Answer from the drawing. Dimensions are ordinates in mm from the lowest x, y and z of the part. A direction names the side the tool comes from. Round coordinates to 2 decimals unless told otherwise and drop trailing zeros. Loops run counter-clockwise (first coordinate to the right, second up) from the corner with the lowest first, then second, coordinate; pieces in that order, holes last. Notation, with made-up numbers: (53.25, 89) - (82.25, 89) arc R9 cw to (82.25, 98) - close; hole circle Ø6 at (53.25, -17). An arc over 180 degrees is marked (long way). Answer as CSV lines item,"result". Start each with the question number.
Q1. Section C-C on z = 6 is taken. Count the separate pieces of the cut face and the enclosed holes in it, then the cut area to 3 significant figures.
Q2. Section D-D on y = 67 is taken. Write down the section's boundary in (x, z).
Q3. For the marked faces 1 and 2, determine the directions among +Z, -Z, +X, -X, +Y, -Y from which every point of the face is accessible in a straight line to the end or side of a thin tool.
Q4. Each of these flat-tipped pins is pushed along its axis until it touches: pin 1 Ø4.5 at (x, y) = (46, 8) entering from +Z; pin 2 Ø15 at (x, y) = (32.5, 38.5) entering from +Z. Where does it stop, or does it pass through?
Q5. The mould has two halves that part along X. Classify the marked faces 3, 4, 5 and 6: +X half, -X half, draft (parallel to the pull), parting line (faces both ways), or undercut.
Q6. Straight lines are drawn through the part: L1, parallel to Y at x = 46, z = 2.5; L2, parallel to Y at x = 27, z = 6.25; L3, parallel to X at y = 73, z = 3. For each, find the intervals that lie inside material, in ascending order. Write a range as [from, to].
Q7. Section B-B on y = 41 is taken. Write down the section's boundary in (x, z).
Q8. Section A-A on x = 8 is taken. Write down the section's boundary in (y, z).
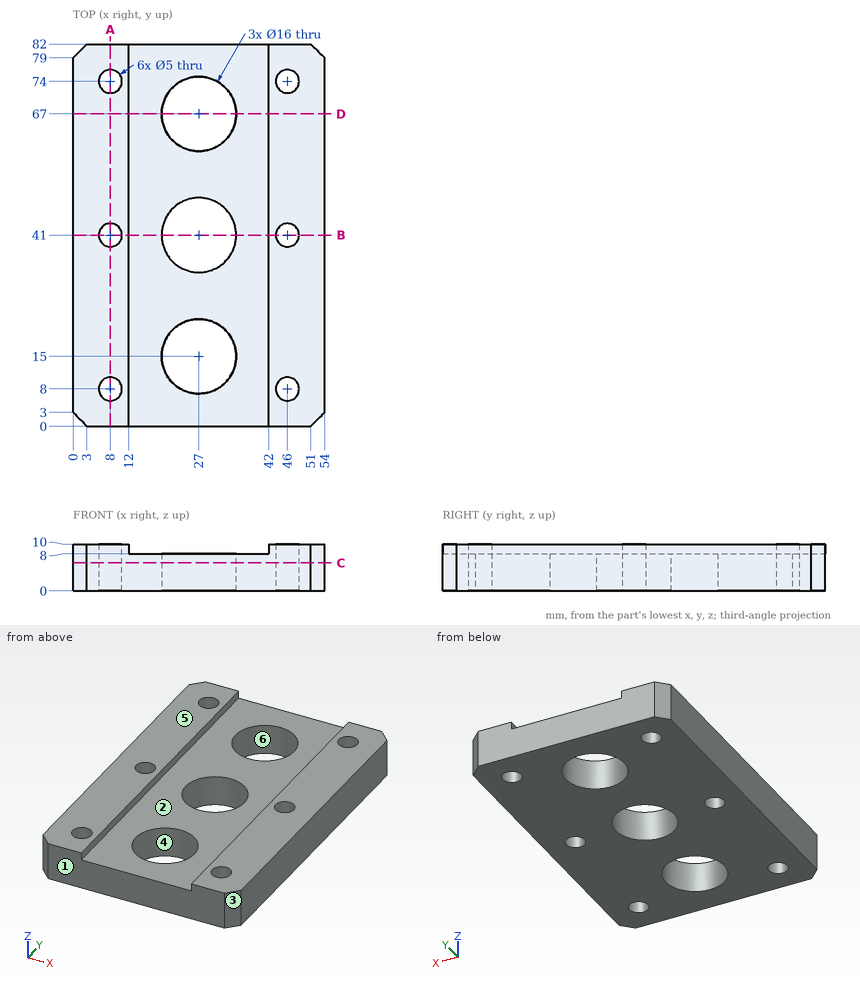
Findings:
1,separate pieces,"1"
1,enclosed holes,"9"
1,area,"3,690 mm^2"
2,outline,"(0, 0) - (19, 0) - (19, 8) - (12, 8) - (12, 10) - (0, 10) - close; (35, 0) - (54, 0) - (54, 10) - (42, 10) - (42, 8) - (35, 8) - close"
3,face 1,"+Z, -Z, +X, -X, -Y"
3,face 2,"+Z, +Y, -Y"
4,pin 1,"passes through"
4,pin 2,"stops at z = 8"
5,face 3,"+X half"
5,face 4,"undercut"
5,face 5,"draft"
5,face 6,"undercut"
6,L1,"y = [0, 5.5], [10.5, 38.5], [43.5, 71.5], [76.5, 82]"
6,L2,"y = [0, 7], [23, 33], [49, 59], [75, 82]"
6,L3,"x = [0, 5.71], [10.29, 21.71], [32.29, 43.71], [48.29, 54]"
7,outline,"(0, 0) - (5.5, 0) - (5.5, 10) - (0, 10) - close; (10.5, 0) - (19, 0) - (19, 8) - (12, 8) - (12, 10) - (10.5, 10) - close; (35, 0) - (43.5, 0) - (43.5, 10) - (42, 10) - (42, 8) - (35, 8) - close; (48.5, 0) - (54, 0) - (54, 10) - (48.5, 10) - close"
8,outline,"(0, 0) - (5.5, 0) - (5.5, 10) - (0, 10) - close; (10.5, 0) - (38.5, 0) - (38.5, 10) - (10.5, 10) - close; (43.5, 0) - (71.5, 0) - (71.5, 10) - (43.5, 10) - close; (76.5, 0) - (82, 0) - (82, 10) - (76.5, 10) - close"
